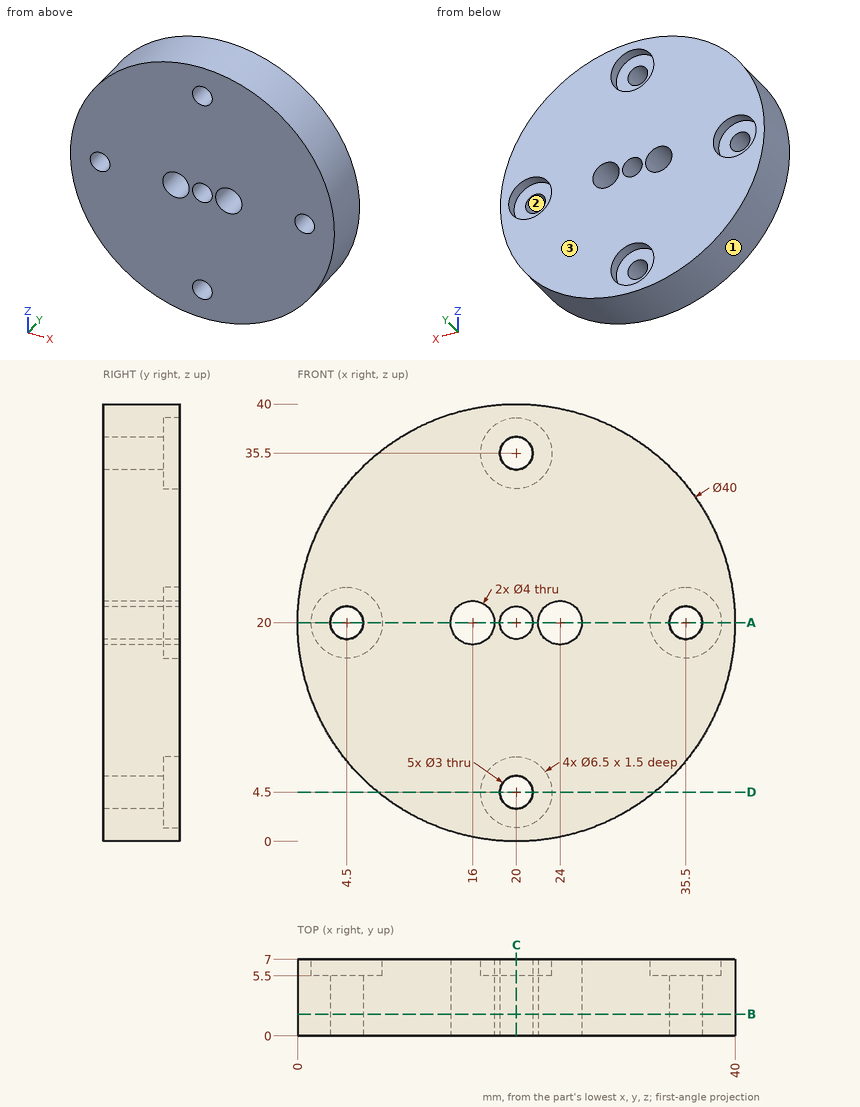
For this review, use the dimensioned drawing (mm, ordinates from the lowest corner) and the shaded views. Round coordinates to 2 decimals unless told otherwise and drop trailing zeros. Order: outer loops, then holes, each group sorted by start corner. A loop starts at its lowest first (then second) coordinate and runs counter-clockwise, first axis right, second up. Notation, with made-up numbers: (38.5, 36.5) -> (71.5, 36.5) arc R22 cw to (71.5, 63.5) -> close; hole circle Ø7 at (88, 0.5). An arc over 180 degrees is marked (long way). One line per item, written item: value. Start each with the question number.
Q1. Wall thickness on line 1 (X direction, y = 3.5, z = 20); line 2 (X direction, y = 6.2, z = 20); line 3 (Y direction, x = 22.5, z = 5): over which ranges is each line inside the solid? List them lowest first.
Q2. Take a section at C-C (x = 20). Write out the cut boundary in (y, z), and give its area (4 significant figures).
Q3. Clearance check with flat-ended pins moving along their axes: pin 1 Ø2 at (x, z) = (34, 19.5) entering from +Y; pin 2 Ø4 at (y, z) = (5.5, 19.5) entering from +X; pin 3 Ø1 at (x, y) = (27.5, 3) entering from -Z (3 decimals). State where each tip first meets the part, or that it passes through.
Q4. Mouldability with a two-part tool opening along Z and no side actions: class the marked faces 1, 2 and 3 as released by +Z, released by -Z, zero draft, split by the parting line, or undercut.
Q5. Take a section at D-D (z = 4.5). Write out the cut boundary in (x, y).
Q6. Take a section at B-B (y = 2). Write out the cut boundary in (x, z).
Q7. Take a section at A-A (z = 20). Count the separate pieces of the cut face and the enclosed holes in it, and give its area (4 significant figures).
Reported:
1. line 1: x = 0 to 3, 6 to 14, 18 to 18.5, 21.5 to 22, 26 to 34, 37 to 40
1. line 2: x = 0 to 1.25, 7.75 to 14, 18 to 18.5, 21.5 to 22, 26 to 32.25, 38.75 to 40
1. line 3: y = 0 to 5.5
2. outline: (0, 0) -> (7, 0) -> (7, 1.25) -> (5.5, 1.25) -> (5.5, 3) -> (0, 3) -> close; (0, 6) -> (5.5, 6) -> (5.5, 7.75) -> (7, 7.75) -> (7, 18.5) -> (0, 18.5) -> close; (0, 21.5) -> (7, 21.5) -> (7, 32.25) -> (5.5, 32.25) -> (5.5, 34) -> (0, 34) -> close; (0, 37) -> (5.5, 37) -> (5.5, 38.75) -> (7, 38.75) -> (7, 40) -> (0, 40) -> close
2. area: 206.5 mm2
3. pin 1: stops at y = 5.5
3. pin 2: stops at x = 40
3. pin 3: stops at z = 1.265
4. face 1: split by the parting line
4. face 2: undercut
4. face 3: zero draft
5. outline: (7.36, 0) -> (18.5, 0) -> (18.5, 5.5) -> (16.75, 5.5) -> (16.75, 7) -> (7.36, 7) -> close; (21.5, 0) -> (32.64, 0) -> (32.64, 7) -> (23.25, 7) -> (23.25, 5.5) -> (21.5, 5.5) -> close
6. outline: circle Ø40 at (20, 20); hole circle Ø3 at (4.5, 20); hole circle Ø4 at (16, 20); hole circle Ø3 at (20, 4.5); hole circle Ø3 at (20, 20); hole circle Ø3 at (20, 35.5); hole circle Ø4 at (24, 20); hole circle Ø3 at (35.5, 20)
7. separate pieces: 6
7. enclosed holes: 0
7. area: 150.5 mm2
